Job drawing, mm, ordinate dimensions from the low corner. One solid piece. Round coordinates to 2 decimals unless told otherwise and drop trailing zeros. Write each loop counter-clockwise with the first axis right and the second up, starting at its lowest first coordinate (ties: lowest second). Pieces come first, ordered by that corner, then holes.
1) Drill centre lines: L1, parallel to Y at x = 70, z = 1; L2, parallel to Y at x = 22, z = 1.9; L3, parallel to Y at x = 33, z = 3.6. Where is each one in solid material? Low to high.
2) Flat gauge pins, fed straight in: pin 1 (3 mm diameter, centred on x = 70, y = 65, fed in from -Z); pin 2 (1.5 mm diameter, centred on y = 3.5, z = 3, fed in from +X). Where does each tip first touch, or does it go through?
3) Saw through at C-C on z = 1.55. Write the cut outline in (x, y).
4) Saw through at B-B on y = 25. Write the cut outline in (x, z), and give its area (3 significant figures).
5) Saw through at D-D on x = 22. Write the cut outline in (y, z).
6) Saw through at A-A on x = 70. Write the cut outline in (y, z), and give its area (4 significant figures).
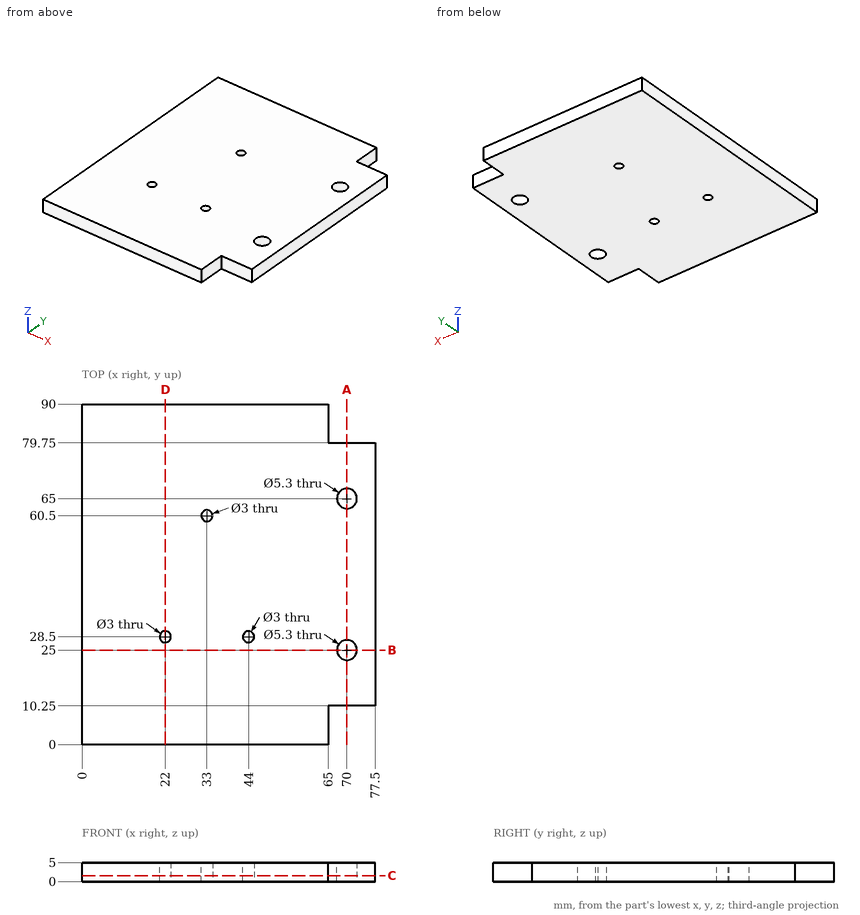
Completed:
1. L1: y = 10.25 to 22.35, 27.65 to 62.35, 67.65 to 79.75
1. L2: y = 0 to 27, 30 to 90
1. L3: y = 0 to 59, 62 to 90
2. pin 1: passes through
2. pin 2: stops at x = 65
3. outline: (0, 0) - (65, 0) - (65, 10.25) - (77.5, 10.25) - (77.5, 79.75) - (65, 79.75) - (65, 90) - (0, 90) - close; hole circle Ø3 at (22, 28.5); hole circle Ø3 at (33, 60.5); hole circle Ø3 at (44, 28.5); hole circle Ø5.3 at (70, 25); hole circle Ø5.3 at (70, 65)
4. outline: (0, 0) - (67.35, 0) - (67.35, 5) - (0, 5) - close; (72.65, 0) - (77.5, 0) - (77.5, 5) - (72.65, 5) - close
4. area: 361 mm2
5. outline: (0, 0) - (27, 0) - (27, 5) - (0, 5) - close; (30, 0) - (90, 0) - (90, 5) - (30, 5) - close
6. outline: (10.25, 0) - (22.35, 0) - (22.35, 5) - (10.25, 5) - close; (27.65, 0) - (62.35, 0) - (62.35, 5) - (27.65, 5) - close; (67.65, 0) - (79.75, 0) - (79.75, 5) - (67.65, 5) - close
6. area: 294.5 mm2
